Build history of the part. All positions in model axes, mm. Face numbers are marked on the shaded views. A direction names the side the tool comes from. Round coordinates to 2 decimals unless told otherwise and drop trailing zeros. Write each loop counter-clockwise with the first axis right and the second up, starting at its lowest first coordinate (ties: lowest second). Pieces come first, ordered by that corner, then holes. Notation, with made-up numbers: (-15, -39.5) - (3, -39.5) arc R17 cw to (3, -12.5) - close; hole circle Ø10 at (-15, -1.5). An arc over 180 degrees is marked (long way). Answer as a JSON object with one key per item and string values. Group by question number.
Item 1: Which spindle directions (+Z, -Z, +X, -X, +Y, -Y) get a long thin tool onto all of the face, cutting with end or side? Do the marked faces 1 and 2. Say none if no direction does.
Item 2: Slice it at A-A, the plane y = 3. List the corners of the cut face in (x, z), then the cut area to 3 significant figures.
Item 3: Probe line 1 (Y direction, x = 8.5, z = -1); line 2 (X direction, y = -16.5, z = -0.25); line 3 (Z direction, x = 3.75, y = 0.5). List the from-to ranges inside material, lowest first. Write a range as from..to.
Item 4: Slice it at C-C, the plane y = -18. List the corners of the cut face in (x, z).
Item 5: Slice it at B-B, the plane z = 0. List the corners of the cut face in (x, y).
Item 6: Flat gauge pins, fed straight in: pin 1 (3 mm diameter, centred on x = -6, z = -8.5, fed in from -Y); pin 2 (1 mm diameter, centred on y = -52, z = 4.5, fed in from -X); pin 3 (12 mm diameter, centred on x = -4.5, y = -52, fed in from -Z). Where does each tip first touch, or does it go through?
from build123d import *

# Parameters (mm, degrees)
BOSS_EXTRUDE1_DEPTH = 10
SKETCH3_R           = 4.5
BOSS_EXTRUDE2_DEPTH = 60
CHAMFER1_SIZE       = 1


with BuildPart() as part:
    # Sketch1 → Boss-Extrude1 (new body)
    with BuildSketch(Plane(origin=(0, 0, 0), x_dir=(1, 0, 0), z_dir=(0, 1, 0))):
        Polygon((10, 5.773502692), (0, 11.547005384), (-10, 5.773502692), (-10, -5.773502692), (0, -11.547005384), (10, -5.773502692), align=None)
    extrude(amount=BOSS_EXTRUDE1_DEPTH)

    # Sketch2 → Cut-Revolve1 (revolve, cut)
    with BuildSketch(Plane(origin=(0, 0, 0), x_dir=(0, 0, -1), z_dir=(1, 0, 0))):
        Polygon((-11.547005384, 10), (-10.047005384, 10), (-11.547005384, 9), align=None)
    revolve(axis=Axis((0, 0, 0), (0, 1, 0)), mode=Mode.SUBTRACT)

    # Sketch3 → Boss-Extrude2 (add)
    with BuildSketch(Plane.XZ):
        with Locations(Location((0, 0, 0), (0, 0, 270))):
            Circle(SKETCH3_R)
    extrude(amount=BOSS_EXTRUDE2_DEPTH)

    # Chamfer1
    chamfer1_edges = [part.edges().sort_by_distance(p)[0] for p in [
        (0, -60, 4.5),
    ]]
    chamfer(chamfer1_edges, length=CHAMFER1_SIZE)


solid = part.part
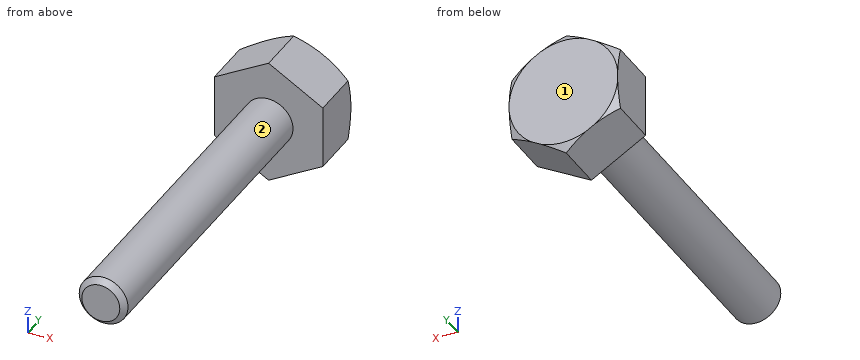
Geometry says:
{
 "1": {"face 1": "+Z, -Z, +X, -X, +Y", "face 2": "-Y"},
 "2": {"outline": "(-10, -5.77) - (0, -11.55) - (10, -5.77) - (10, 5.77) - (0, 11.55) - (-10, 5.77) - close", "area": "346 mm^2"},
 "3": {"line 1": "y = 0..10", "line 2": "x = -4.49..4.49", "line 3": "z = -9.38..9.38"},
 "4": {"outline": "circle Ø9 at (0, 0)"},
 "5": {"outline": "(-10, 0) - (-4.5, 0) - (-4.5, -59) - (-3.5, -60) - (3.5, -60) - (4.5, -59) - (4.5, 0) - (10, 0) - (10, 10) - (-10, 10) - close"},
 "6": {"pin 1": "stops at y = 0", "pin 2": "stops at x = -2.06", "pin 3": "stops at z = -4.5"}
}
